```python
from build123d import *

# Parameters (mm, degrees)
F0_R         = 3.7
F1_DEPTH     = 17
F2_T1_DEPTH  = 81.7
F2_T3_DEPTH  = 8
F2_T6_ANGLE  = 90
F2_T8_ANGLE  = 90
F2_T10_ANGLE = 90
F2_T12_ANGLE = 90


# Not quite as in the source:
# - a fillet or chamfer that OpenCascade refuses, or shapes differently, is made with other operations: its cross-section is extruded or revolved along the edge and cut away or added


with BuildPart() as f1:
    # F0 (on Top) → F1 (new body)
    with BuildSketch(Plane.XY):
        with BuildLine():
            ThreePointArc((-4.5, -4), (-4.2071067812, -4.7071067812), (-3.5, -5))
            Line((-3.5, -5), (78.2, -5))
            ThreePointArc((78.2, -5), (78.9071067812, -4.7071067812), (79.2, -4))
            Line((79.2, -4), (79.2, 4))
            ThreePointArc((79.2, 4), (78.9071067812, 4.7071067812), (78.2, 5))
            Line((78.2, 5), (-3.5, 5))
            ThreePointArc((-3.5, 5), (-4.2071067812, 4.7071067812), (-4.5, 4))
            Line((-4.5, 4), (-4.5, -4))
        make_face()
        Circle(F0_R, mode=Mode.SUBTRACT)
        with Locations((8.3, 0)):
            Circle(F0_R, mode=Mode.SUBTRACT)
        with Locations((16.6, 0)):
            Circle(F0_R, mode=Mode.SUBTRACT)
        with Locations((24.9, 0)):
            Circle(F0_R, mode=Mode.SUBTRACT)
        with Locations((33.2, 0)):
            Circle(F0_R, mode=Mode.SUBTRACT)
        with Locations((41.5, 0)):
            Circle(F0_R, mode=Mode.SUBTRACT)
        with Locations((49.8, 0)):
            Circle(F0_R, mode=Mode.SUBTRACT)
        with Locations((58.1, 0)):
            Circle(F0_R, mode=Mode.SUBTRACT)
        with Locations((66.4, 0)):
            Circle(F0_R, mode=Mode.SUBTRACT)
        with Locations((74.7, 0)):
            Circle(F0_R, mode=Mode.SUBTRACT)
    extrude(amount=F1_DEPTH)

    # F2: fillet of radius 1 on 8 edges, made by hand

    # F2_s2 → F2_t1 (cut)
    with BuildSketch(Plane.YZ.offset(-3.5)):
        with BuildLine():
            ThreePointArc((-5, 16), (-4.7071067812, 16.7071067812), (-4, 17))
            Line((-4, 17), (-5, 17))
            Line((-5, 17), (-5, 16))
        make_face()
        with BuildLine():
            ThreePointArc((5, 16), (4.7071067812, 16.7071067812), (4, 17))
            Line((4, 17), (5, 17))
            Line((5, 17), (5, 16))
        make_face()
    extrude(amount=F2_T1_DEPTH, mode=Mode.SUBTRACT)

    # F2_s4 → F2_t3 (cut)
    with BuildSketch(Plane.XZ.offset(-4)):
        with BuildLine():
            ThreePointArc((79.2, 16), (78.9071067812, 16.7071067812), (78.2, 17))
            Line((78.2, 17), (79.2, 17))
            Line((79.2, 17), (79.2, 16))
        make_face()
        with BuildLine():
            ThreePointArc((-4.5, 16), (-4.2071067812, 16.7071067812), (-3.5, 17))
            Line((-3.5, 17), (-4.5, 17))
            Line((-4.5, 17), (-4.5, 16))
        make_face()
    extrude(amount=F2_T3_DEPTH, mode=Mode.SUBTRACT)

    # F2_s5 → F2_t6 (revolve, cut)
    with BuildSketch(Plane.XZ.offset(4)):
        with BuildLine():
            ThreePointArc((-4.5, 16), (-4.2071067812, 16.7071067812), (-3.5, 17))
            Line((-3.5, 17), (-4.5, 17))
            Line((-4.5, 17), (-4.5, 16))
        make_face()
    revolve(axis=Axis((-3.5, -4, 17), (0, 0, 1)), revolution_arc=F2_T6_ANGLE, mode=Mode.SUBTRACT)

    # F2_s7 → F2_t8 (revolve, cut)
    with BuildSketch(Plane.YZ.offset(78.2)):
        with BuildLine():
            ThreePointArc((-5, 16), (-4.7071067812, 16.7071067812), (-4, 17))
            Line((-4, 17), (-5, 17))
            Line((-5, 17), (-5, 16))
        make_face()
    revolve(axis=Axis((78.2, -4, 17), (0, 0, 1)), revolution_arc=F2_T8_ANGLE, mode=Mode.SUBTRACT)

    # F2_s9 → F2_t10 (revolve, cut)
    with BuildSketch(Plane.XZ.offset(-4)):
        with BuildLine():
            ThreePointArc((79.2, 16), (78.9071067812, 16.7071067812), (78.2, 17))
            Line((78.2, 17), (79.2, 17))
            Line((79.2, 17), (79.2, 16))
        make_face()
    revolve(axis=Axis((78.2, 4, 17), (0, 0, 1)), revolution_arc=F2_T10_ANGLE, mode=Mode.SUBTRACT)

    # F2_s11 → F2_t12 (revolve, cut)
    with BuildSketch(Plane.YZ.offset(-3.5)):
        with BuildLine():
            ThreePointArc((5, 16), (4.7071067812, 16.7071067812), (4, 17))
            Line((4, 17), (5, 17))
            Line((5, 17), (5, 16))
        make_face()
    revolve(axis=Axis((-3.5, 4, 17), (0, 0, 1)), revolution_arc=F2_T12_ANGLE, mode=Mode.SUBTRACT)


solid = f1.part
```
The listing builds one solid part. Answer for the finished solid, in the listing's coordinates (mm). Round coordinates to 2 decimals unless told otherwise and drop trailing zeros. Write each loop counter-clockwise with the first axis right and the second up, starting at its lowest first coordinate (ties: lowest second). Pieces come first, ordered by that corner, then holes. Notation, with made-up numbers: (49, -35.5) -> (101, -35.5) arc R23 cw to (101, -5.5) -> close; hole circle Ø6 at (-2.75, 30.25). An arc over 180 degrees is marked (long way). Answer as a JSON object with one key per item and string values. Group by question number.
Q1. Straight lines are drawn through the part: line 1 along Y through (x, z) = (16.6, 8.5); line 2 along Y through (x, z) = (19.5, 14.5); line 3 along X through (y, z) = (4.75, 12.25). For each, find the intervals that lie inside material, in ascending order.
Q2. Section B-B (z = 5.5) is taken. Count the separate pieces of the cut face and the enclosed holes in it, plus the area to 3 significant figures.
Q3. Section D-D (x = 63.5) is taken. Write down the section's boundary in (y, z), plus the area to 3 significant figures.
Q4. Section A-A (x = 41.5) is taken. Write down the section's boundary in (y, z), plus the area to 3 significant figures.
Q5. Determine the mould class of faces 1 (the face through (37, -5, 8)), 2 (the face through (-0.802, -3.612, 8.381)), 3 (the face through (37, 1, 0)) for opening direction Y: pulls with the +Y half, pulls with the -Y half, needs draft (parallel to the pull), parting line crosses it, or undercut.
Check values:
{
 "1": {"line 1": "-5 to -3.7, 3.7 to 5", "line 2": "-5 to -2.3, 2.3 to 5", "line 3": "-4.16 to 78.86"},
 "2": {"separate pieces": "1", "enclosed holes": "10", "area": "406 mm^2"},
 "3": {"outline": "(-5, 0) -> (-2.3, 0) -> (-2.3, 17) -> (-4, 17) arc R1 ccw to (-5, 16) -> close; (2.3, 0) -> (5, 0) -> (5, 16) arc R1 ccw to (4, 17) -> (2.3, 17) -> close", "area": "91.4 mm^2"},
 "4": {"outline": "(-5, 0) -> (-3.7, 0) -> (-3.7, 17) -> (-4, 17) arc R1 ccw to (-5, 16) -> close; (3.7, 0) -> (5, 0) -> (5, 16) arc R1 ccw to (4, 17) -> (3.7, 17) -> close", "area": "43.8 mm^2"},
 "5": {"face 1": "pulls with the -Y half", "face 2": "undercut", "face 3": "needs draft"}
}
